```python
from build123d import *

# Parameters (mm, degrees)
BOSS_EXTRUDE1_DEPTH        = 15
F_3_5_3_5_DIAMETER_HOLE1_D = 3.5
FILLET1_R                  = 2
F_2_2_2_2_DIAMETER_HOLE1_D = 2.2
CHAMFER1_SIZE              = 1
CHAMFER2_SIZE              = 1


with BuildPart() as part:
    # Sketch1 → Boss-Extrude1 (new, symmetric)
    with BuildSketch(Plane(origin=(0, 0, 0), x_dir=(0, 0, -1), z_dir=(1, 0, 0))):
        Polygon((-15, 0), (15, 0), (15, 3), (0, 3), (0, 13), (-5, 13), (-5, 3), (-15, 3), align=None)
    extrude(amount=BOSS_EXTRUDE1_DEPTH, both=True)

    # Ø3.5 (3.5) Diameter Hole1 (through all)
    with Locations(Plane(origin=(0, 3, 0), x_dir=(1, 0, 0), z_dir=(0, 1, 0))):
        with Locations((-12.02948497, 12), (12.02948497, 12), (-12.02948497, -12), (12.02948497, -12)):
            Hole(F_3_5_3_5_DIAMETER_HOLE1_D / 2)

    # Fillet1
    fillet1_edges = [part.edges().sort_by_distance(p)[0] for p in [
        (-15, 1.5, -15),
        (15, 1.5, 15),
        (15, 1.5, -15),
        (-15, 1.5, 15),
    ]]
    fillet(fillet1_edges, radius=FILLET1_R)

    # Ø2.2 (2.2) Diameter Hole1 (through all)
    with Locations(Plane(origin=(0, 0, 0), x_dir=(-1, 0, 0), z_dir=(0, 0, -1))):
        with Locations((-10, 6), (10, 6)):
            Hole(F_2_2_2_2_DIAMETER_HOLE1_D / 2)

    # Chamfer1
    chamfer1_edges = [part.edges().sort_by_distance(p)[0] for p in [
        (0, 3, 5),
        (0, 3, 0),
    ]]
    chamfer(chamfer1_edges, length=CHAMFER1_SIZE)

    # Chamfer2
    chamfer2_edges = [part.edges().sort_by_distance(p)[0] for p in [
        (-15, 13, 2.5),
        (15, 13, 2.5),
    ]]
    chamfer(chamfer2_edges, length=CHAMFER2_SIZE)


solid = part.part
```
The listing builds one solid part. Answer for the finished solid, in the listing's coordinates (mm). A direction names the side the tool comes from. Give positions to 0.01 mm unless a question says otherwise; leave off trailing zeros. Order: outer loops, then holes, each group sorted by start corner. A loop starts at its lowest first (then second) coordinate and runs counter-clockwise, first axis right, second up.
Item 1: The part is cut by section C-C, the plane z = 0.75. Give the vertices of the cut face in (x, y).
From the geometry:
outline: (-15, 0) - (15, 0) - (15, 12) - (14, 13) - (-14, 13) - (-15, 12) - close; hole circle Ø2.2 at (-10, 6); hole circle Ø2.2 at (10, 6)
Item 2: The part is cut by section A-A, the plane z = 12. Give the vertices of the cut face in (x, y), and give its area (3 significant figures).
From the geometry:
outline: (-15, 0) - (-13.78, 0) - (-13.78, 3) - (-15, 3) - close; (-10.28, 0) - (10.28, 0) - (10.28, 3) - (-10.28, 3) - close; (13.78, 0) - (15, 0) - (15, 3) - (13.78, 3) - close
area: 69.0 mm2
Item 3: For a pull along Y with two mould halves and no side action, classify faces 4 (the face through (0, 3, 10)), 5 (the face through (11.05, 6.33, 2.54)), 6 (the face through (0, 8, 0)), 7 (the face through (-8.95, 6.33, 2.54)) as pulls with the +Y half, pulls with the -Y half, needs draft (parallel to the pull), parting line crosses it, or undercut.
From the geometry:
face 4: pulls with the +Y half
face 5: undercut
face 6: needs draft
face 7: undercut
Item 4: Given pin 1 Ø7 at (x, z) = (-1.5, -8) entering from +Y; pin 2 Ø2 at (x, z) = (-12.03, -12) entering from +Y; pin 3 Ø1 at (x, y) = (-2, 8) entering from -Z; pin 4 Ø7 at (x, y) = (-5, 10) entering from +Z, each flat-ended and moving along its own axis, determine where each tip first touches the part or whether it passes through.
From the geometry:
pin 1: stops at y = 3
pin 2: passes through
pin 3: stops at z = 0
pin 4: stops at z = 5
Item 5: Find the intervals of material crossed by probe 1 along X at (y, z) = (1.5, 12); probe 2 along Z at (x, y) = (0.25, 8.5); probe 3 along Y at (x, z) = (13.75, 8.25), in increasing order.
From the geometry:
probe 1: x = -15 to -13.78, -10.28 to 10.28, 13.78 to 15
probe 2: z = 0 to 5
probe 3: y = 0 to 3
Item 6: The part is cut by section B-B, the plane y = 2.5. Give the vertices of the cut face in (x, z).
From the geometry:
outline: (-15, -13) arc R2 ccw to (-13, -15) - (13, -15) arc R2 ccw to (15, -13) - (15, 13) arc R2 ccw to (13, 15) - (-13, 15) arc R2 ccw to (-15, 13) - close; hole circle Ø3.5 at (-12.03, -12); hole circle Ø3.5 at (-12.03, 12); hole circle Ø3.5 at (12.03, -12); hole circle Ø3.5 at (12.03, 12)
Item 7: The part is cut by section D-D, the plane x = 1.75. Give the vertices of the cut face in (y, z).
From the geometry:
outline: (0, -15) - (3, -15) - (3, -1) - (4, 0) - (13, 0) - (13, 5) - (4, 5) - (3, 6) - (3, 15) - (0, 15) - close
Item 8: Which of the six approach directions +Z, -Z, +X, -X, +Y, -Y give full straight-line access (tool end or side, diameter ignored) to faces 1 (the face through (-11.802, 1.479, -13.735)), 2 (the face through (0, 3, -8)), 3 (the face through (0, 9, 5))?
From the geometry:
face 1: +Y, -Y
face 2: -Z, +X, -X, +Y
face 3: +Z, +X, -X, +Y
